For this review, take the finished solid that the model builds, in its own axes (mm). Face numbers are marked on the shaded views. A direction names the side the tool comes from. Coordinates: 2 decimals unless noted, no trailing zeros. Order: outer loops, then holes, each group sorted by start corner. A loop starts at its lowest first (then second) coordinate and runs counter-clockwise, first axis right, second up. Notation, with made-up numbers: (44, 2.5) -> (76, 2.5) arc R11 ccw to (76, 11.5) -> close; hole circle Ø8 at (-10, -7.5). An arc over 180 degrees is marked (long way). Answer as a JSON object with one key per item and string values. Group by question number.
1) Add section C-C, the plane y = 10. Write out the cut boundary in (x, z), then the cut area to 3 significant figures.
2) Add section B-B, the plane x = 0. Write out the cut boundary in (y, z) (3 decimals).
3) Draft analysis for pull direction X (two halves, no side actions). For the marked faces 4, 5 and 6, state which applies: +X half, -X half, draft (parallel to the pull), parting line (faces both ways), or undercut.
4) Add section D-D, the plane z = 0. Write out the cut boundary in (x, y) (3 decimals), then the cut area to 3 significant figures.
5) Wall thickness on L1, parallel to X at y = 2.2, z = 0; L2, parallel to X at y = 7.5, z = 0; L3, parallel to Z at x = 0.25, y = 11.5: over which ranges is each line inside the solid? List them lowest first.
6) For pin 1 (1.5 mm diameter, centred on y = -2.5, z = -5, fed in from -X); pin 2 (6 mm diameter, centred on x = 1.5, y = -8.5, fed in from +Z); pin 3 (4.5 mm diameter, centred on x = -1.5, z = 2, fed in from +Y); pin 4 (3 mm diameter, centred on x = -5.5, z = 3.5, fed in from -Y), all flat-tipped, find the tip position at first contact; note any pin that passes through.
7) Add section A-A, the plane y = 13.5. Write out the cut boundary in (x, z), then the cut area to 3 significant figures.
8) Machinability: for the marked faces 1, 2 and 3, which of the approach directions +Z, -Z, +X, -X, +Y, -Y give a long, thin tool a straight path to every point of the face, cutting with its end or side? Answer none if there is none.
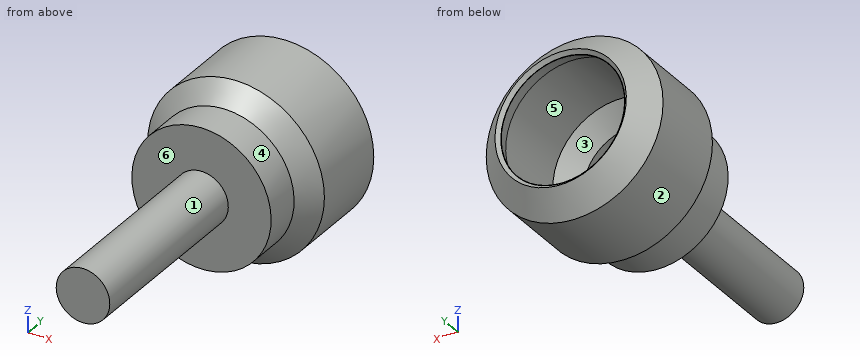
from build123d import *

# Parameters (mm, degrees)
SKETCH2_R           = 2.5
BOSS_EXTRUDE1_DEPTH = 18


with BuildPart() as part:
    # Sketch1 → Revolve1 (revolve)
    with BuildSketch(Plane.XY, mode=Mode.PRIVATE) as revolve1_sk:
        Polygon((0, 0), (-6.5, 0), (-6.5, 3.48875), (-8.25, 5.23875), (-8.25, 12.73875), (-6.128679656, 14.860070344), (-5.790903941, 14.522294629), (-7.75, 12.56319857), (-7.75, 5.56319857), (-6, 3.81319857), (-6, 0.5), (0, 0.5), align=None)
    revolve(revolve1_sk.sketch.rotate(Axis((0, 0.5, 0), (0, -1, 0)), 270), axis=Axis((0, 0.5, 0), (0, -1, 0)))

    # Sketch2 → Boss-Extrude1 (add)
    with BuildSketch(Plane.XZ):
        with Locations(Location((0, 0, 0), (0, 0, 270))):
            Circle(SKETCH2_R)
    extrude(amount=BOSS_EXTRUDE1_DEPTH)

    # Sketch3 → Revolve2 (revolve)
    with BuildSketch(Plane.XY, mode=Mode.PRIVATE) as revolve2_sk:
        Polygon((7.756571399, 12.572177682), (7.756571399, 5.526763194), (6.042904197, 3.762081274), (6.042904197, 0.47971139), (0, 0.47971139), (0, 1.150787733), (4.526358004, 1.150787733), (4.526358004, 4.087737861), (6.256571399, 5.869458543), (6.256571399, 12.21791401), (6.256571399, 13.029033499), (5.755922464, 14.51499039), align=None)
    revolve(revolve2_sk.sketch.rotate(Axis((0, 0.47971139, 0), (0, 1, 0)), 90), axis=Axis((0, 0.47971139, 0), (0, 1, 0)))


solid = part.part
Output values:
{
 "1": {"outline": "circle Ø16.5 at (0, 0); hole circle Ø12.51 at (0, 0)", "area": "90.8 mm²"},
 "2": {"outline": "(-18, -2.5) -> (0, -2.5) -> (0, -6.5) -> (3.489, -6.5) -> (5.239, -8.25) -> (12.739, -8.25) -> (14.86, -6.129) -> (14.522, -5.791) -> (13.095, -7.219) -> (14.515, -5.756) -> (13.029, -6.257) -> (5.869, -6.257) -> (4.088, -4.526) -> (1.151, -4.526) -> (1.151, 4.526) -> (4.088, 4.526) -> (5.869, 6.257) -> (13.029, 6.257) -> (14.515, 5.756) -> (13.095, 7.219) -> (14.522, 5.791) -> (14.86, 6.129) -> (12.739, 8.25) -> (5.239, 8.25) -> (3.489, 6.5) -> (0, 6.5) -> (0, 2.5) -> (-18, 2.5) -> close"},
 "3": {"face 4": "parting line", "face 5": "undercut", "face 6": "draft"},
 "4": {"outline": "(-8.25, 5.239) -> (-6.5, 3.489) -> (-6.5, 0) -> (-2.5, 0) -> (-2.5, -18) -> (2.5, -18) -> (2.5, 0) -> (6.5, 0) -> (6.5, 3.489) -> (8.25, 5.239) -> (8.25, 12.739) -> (6.129, 14.86) -> (5.791, 14.522) -> (7.219, 13.095) -> (5.756, 14.515) -> (6.257, 13.029) -> (6.257, 5.869) -> (4.526, 4.088) -> (4.526, 1.151) -> (-4.526, 1.151) -> (-4.526, 4.088) -> (-6.257, 5.869) -> (-6.257, 13.029) -> (-5.756, 14.515) -> (-7.219, 13.095) -> (-5.791, 14.522) -> (-6.129, 14.86) -> (-8.25, 12.739) -> close", "area": "158 mm²"},
 "5": {"L1": "x = -6.5 to -4.53, 4.53 to 6.5", "L2": "x = -8.25 to -6.26, 6.26 to 8.25", "L3": "z = -8.25 to -6.25, 6.25 to 8.25"},
 "6": {"pin 1": "passes through", "pin 2": "stops at z = 2.5", "pin 3": "stops at y = 4.32", "pin 4": "stops at y = 0"},
 "7": {"outline": "circle Ø14.98 at (0, 0); circle Ø13.6 at (0, 0); hole circle Ø13.63 at (0, 0); hole circle Ø12.2 at (0, 0)", "area": "58.9 mm²"},
 "8": {"face 1": "-Y", "face 2": "+Y, -Y", "face 3": "none"}
}
